CAD build for the part. Positions are in the model's coordinates, mm. A direction names the side the tool comes from. Coordinates: 2 decimals unless noted, no trailing zeros. Loops run counter-clockwise (first coordinate to the right, second up) from the corner with the lowest first, then second, coordinate; pieces in that order, holes last. Notation, with made-up numbers: M 71,13 L 107,13 A8 ccw 107,21 Z; hole C 35.5,47 d5. An arc over 180 degrees is marked long. Answer as a JSON object with one key per item and string values. Group by question number.
```python
from build123d import *

# Parameters (mm, degrees)
SKETCH1_R           = 3.1496
BOSS_EXTRUDE1_DEPTH = 14.2875
SKETCH3_R           = 3.1496
SKETCH3_R_2         = 2.3876
CUT_EXTRUDE2_DEPTH  = 7.9375


with BuildPart() as part:
    # Sketch1 → Boss-Extrude1 (new, symmetric)
    with BuildSketch(Plane(origin=(0, 0, 0), x_dir=(0, 0, -1), z_dir=(1, 0, 0))):
        Circle(SKETCH1_R)
    extrude(amount=BOSS_EXTRUDE1_DEPTH, both=True)

    # Sketch3 → Cut-Extrude2 (cut)
    with BuildSketch(Plane(origin=(14.2875, 0, 0), x_dir=(0, 0, -1), z_dir=(1, 0, 0))):
        Circle(SKETCH3_R)
        Circle(SKETCH3_R_2, mode=Mode.SUBTRACT)
    cut_extrude2 = extrude(amount=-CUT_EXTRUDE2_DEPTH, mode=Mode.SUBTRACT)

    # Mirror1: Cut-Extrude2 across plane
    add(cut_extrude2.mirror(Plane(origin=(0, 0, 0), x_dir=(0, 0, 1), z_dir=(1, 0, 0))), mode=Mode.SUBTRACT)


solid = part.part
```
Item 1: Slice it at C-C, the plane x = -7. Write the cut outline in (y, z).
Item 2: Slice it at D-D, the plane x = -2.75. Write the cut outline in (y, z).
Item 3: Slice it at B-B, the plane z = 0.5. Write the cut outline in (x, y), then the cut area to 3 significant figures.
Item 4: Slice it at A-A, the plane y = 0. Write the cut outline in (x, z).
Item 5: Tool access for faces 1 (the flat face through (6.35, 2, 2)), 2 (the cylindrical face through (0.089, -1.916, 2.499)), 3 (the flat face through (-6.35, 2, 2)): list every direction of +Z, -Z, +X, -X, +Y, -Y with a clear straight run to the whole face (end or side of a thin tool).
Item 6: Pin check, flat tips, straight feed: pin 1 (1.5 mm diameter, centred on x = 7.5, z = -0.5, fed in from +Y); pin 2 (2 mm diameter, centred on x = 6.5, y = -2.5, fed in from -Z); pin 3 (3 mm diameter, centred on x = 3.5, y = -2.5, fed in from -Z). Stop position of each tip, or through.
Item 7: Drill centre lines: L1, parallel to X at y = 2.5, z = 0.5; L2, parallel to Y at x = -10.5, z = 0; L3, parallel to Z at x = -3.25, y = 2.25. Where is each one in solid material? Low to high. Write a range as from..to.
Computed:
{
 "1": {"outline": "C 0,0 d4.78"},
 "2": {"outline": "C 0,0 d6.3"},
 "3": {"outline": "M -14.29,-2.33 L -6.35,-2.33 L -6.35,-3.11 L 6.35,-3.11 L 6.35,-2.33 L 14.29,-2.33 L 14.29,2.33 L 6.35,2.33 L 6.35,3.11 L -6.35,3.11 L -6.35,2.33 L -14.29,2.33 Z", "area": "153 mm2"},
 "4": {"outline": "M -14.29,-2.39 L -6.35,-2.39 L -6.35,-3.15 L 6.35,-3.15 L 6.35,-2.39 L 14.29,-2.39 L 14.29,2.39 L 6.35,2.39 L 6.35,3.15 L -6.35,3.15 L -6.35,2.39 L -14.29,2.39 Z"},
 "5": {"face 1": "+X", "face 2": "+X, -X", "face 3": "-X"},
 "6": {"pin 1": "y = 2.39", "pin 2": "z = -2.76", "pin 3": "z = -2.99"},
 "7": {"L1": "-6.35..6.35", "L2": "-2.39..2.39", "L3": "-2.2..2.2"}
}
